Check sheet for the modelled part. Datum: model origin and axes. Units: mm. A direction names the side the tool comes from. Give positions to 0.01 mm unless a question says otherwise; leave off trailing zeros. Write each loop counter-clockwise with the first axis right and the second up, starting at its lowest first coordinate (ties: lowest second). Pieces come first, ordered by that corner, then holes. Notation, with made-up numbers: (9.25, 5) -> (19.25, 5) arc R21 ccw to (19.25, 9) -> close; hole circle Ø3 at (84, 70.5). An arc over 180 degrees is marked (long way). Return JSON: item names as keys, results as strings.
from build123d import *

# Parameters (mm, degrees)
SKETCH1_R           = 26.5
BOSS_EXTRUDE1_DEPTH = 56
SKETCH4_R           = 37.5
BOSS_EXTRUDE2_DEPTH = 5
SKETCH5_R           = 10
CUT_EXTRUDE1_DEPTH  = 81.830068663
CUT_EXTRUDE2_DEPTH  = 5


with BuildPart() as part:
    # Sketch1 → Boss-Extrude1 (new body)
    with BuildSketch(Plane.XY):
        Circle(SKETCH1_R)
    extrude(amount=BOSS_EXTRUDE1_DEPTH)

    # Sketch4 → Boss-Extrude2 (add)
    with BuildSketch(Plane(origin=(0, 0, 0), x_dir=(-1, 0, 0), z_dir=(0, 0, -1))):
        Circle(SKETCH4_R)
    extrude(amount=BOSS_EXTRUDE2_DEPTH)

    # Sketch5 → Cut-Extrude1 (cut, through all)
    with BuildSketch(Plane.XY.offset(56)):
        Circle(SKETCH5_R)
    extrude(amount=-CUT_EXTRUDE1_DEPTH, mode=Mode.SUBTRACT)

    # Sketch6 → Cut-Extrude2 (cut, symmetric)
    with BuildSketch(Plane(origin=(0, 0, 0), x_dir=(1, 0, 0), z_dir=(0, 1, 0))):
        Polygon((20, -29), (18.5, -30.5), (18.5, -35), (20, -36.5), (20, -53), (17, -56), (20, -56), (26.5, -56), (26.5, -29), align=None)
    cut_extrude2 = extrude(amount=CUT_EXTRUDE2_DEPTH, both=True, mode=Mode.SUBTRACT)

    # Mirror1: Cut-Extrude2 across plane
    add(cut_extrude2.mirror(Plane(origin=(0, 0, 0), x_dir=(0, 0, 1), z_dir=(1, 0, 0))), mode=Mode.SUBTRACT)


solid = part.part
(1) Depth check by flat-ended pin: pin 1 Ø5 at (x, y) = (-21.5, 1.5) entering from +Z; pin 2 Ø2.5 at (x, z) = (-19.5, 36) entering from -Y; pin 3 Ø1.3 at (y, z) = (1, 33.5) entering from +X. Enter the tip coordinate at first touch or a pass-through.
Reply:
{"pin 1": "z = 54", "pin 2": "y = -19.21", "pin 3": "x = 18.5"}
(2) Cross-section at D-D on z = 34. Enter the section's corners in (x, y).
Reply:
{"outline": "(-26.02, -5) arc R26.5 ccw to (26.02, -5) -> (18.5, -5) -> (18.5, 5) -> (26.02, 5) arc R26.5 ccw to (-26.02, 5) -> (-18.5, 5) -> (-18.5, -5) -> close; hole circle Ø20 at (0, 0)"}
(3) Thickness scan on L1, parallel to Y at x = 0, z = 38; L2, parallel to X at y = 0.5, z = 45; L3, parallel to Z at x = -4, y = -28. Record the ranges inside material, lowest first.
Reply:
{"L1": "-26.5 to -10, 10 to 26.5", "L2": "-20 to -9.99, 9.99 to 20", "L3": "-5 to 0"}
(4) Cross-section at C-C on x = 0. Enter the section's corners in (y, z), then the cut area to 3 significant figures.
Reply:
{"outline": "(-37.5, -5) -> (-10, -5) -> (-10, 56) -> (-26.5, 56) -> (-26.5, 0) -> (-37.5, 0) -> close; (10, -5) -> (37.5, -5) -> (37.5, 0) -> (26.5, 0) -> (26.5, 56) -> (10, 56) -> close", "area": "2,120 mm^2"}
(5) Cross-section at A-A on z = 46.5. Enter the section's corners in (x, y).
Reply:
{"outline": "(-26.02, -5) arc R26.5 ccw to (26.02, -5) -> (20, -5) -> (20, 5) -> (26.02, 5) arc R26.5 ccw to (-26.02, 5) -> (-20, 5) -> (-20, -5) -> close; hole circle Ø20 at (0, 0)"}
(6) Set-up check for faces 1 (the flat face through (-18.5, 0, 33)), 2 (the cylindrical face through (25.276, 7.96, 27.608)), 3 (the flat face through (20, 0, 45)), 4 (the flat face through (-19, 0, 54)): record each of +Z, -Z, +X, -X, +Y, -Y from which the full face is reachable in a straight line by a thin tool's end or side.
Reply:
{"face 1": "-X", "face 2": "+Z", "face 3": "+Z, +X", "face 4": "+Z, -X"}
(7) Release check for a two-part mould opening along X. For faces 5 (the cylindrical face through (-2.17, -9.76, 25.93)), 6 (the flat face through (-20, 0, 45)), 7 (the flat face through (22, 5, 42)) record: pulls with the +X half, pulls with the -X half, needs draft (parallel to the pull), parting line crosses it, or undercut.
Reply:
{"face 5": "undercut", "face 6": "pulls with the -X half", "face 7": "needs draft"}
(8) Cross-section at B-B on y = 0. Enter the section's corners in (x, z).
Reply:
{"outline": "(-37.5, -5) -> (-10, -5) -> (-10, 56) -> (-17, 56) -> (-20, 53) -> (-20, 36.5) -> (-18.5, 35) -> (-18.5, 30.5) -> (-20, 29) -> (-26.5, 29) -> (-26.5, 0) -> (-37.5, 0) -> close; (10, -5) -> (37.5, -5) -> (37.5, 0) -> (26.5, 0) -> (26.5, 29) -> (20, 29) -> (18.5, 30.5) -> (18.5, 35) -> (20, 36.5) -> (20, 53) -> (17, 56) -> (10, 56) -> close"}
